Read the model definition and answer for the solid it produces. Units are mm, in the model's axes. Face numbers are marked on the shaded views. Coordinates: 2 decimals unless noted, no trailing zeros. Put each result on its own line as item: value.
from build123d import *

# Parameters (mm, degrees)
F0_W     = 600
F0_H     = 800
F1_DEPTH = 150
F2_R     = 30


with BuildPart() as f1:
    # F0 (on Top) → F1 (new body)
    with BuildSketch(Plane.XY):
        Rectangle(F0_W, F0_H)
    extrude(amount=-F1_DEPTH)

    # F2
    f2_edges = [f1.edges().sort_by_distance(p)[0] for p in [
        (300, 400, -75),
        (-300, 400, -75),
        (0, 400, 0),
        (0, 400, -150),
        (-300, -400, -75),
        (-300, 0, 0),
        (-300, 0, -150),
        (0, -400, 0),
        (300, 0, 0),
        (300, -400, -75),
        (0, -400, -150),
        (300, 0, -150),
    ]]
    fillet(f2_edges, radius=F2_R)


solid = f1.part
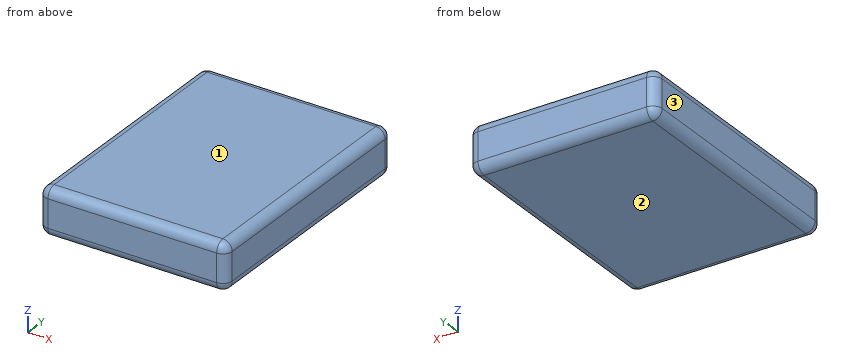
Q1. For a pull along Z with two mould halves and no side action, classify the marked faces 1, 2 and 3 as +Z half, -Z half, draft (parallel to the pull), parting line (faces both ways), or undercut.
Answers below:
face 1: +Z half
face 2: -Z half
face 3: draft
Q2. Given pin 1 (12 mm diameter, centred on x = -55, y = 221, fed in from +Z), flat-ended and moving along its own axis, determine where the tip first touches the part or whether it passes through.
Answers below:
pin 1: stops at z = 0
Q3. Consider line 1 along Y through (x, z) = (69.5, -27.5); line 2 along Y through (x, z) = (149, -7); line 3 along X through (y, z) = (-103.5, -8). Determine where each line is inside the solid, lowest interval first.
Answers below:
line 1: y = -399.9 to 399.9
line 2: y = -389.26 to 389.26
line 3: x = -290.4 to 290.4
